from build123d import *

# Parameters (mm, degrees)
ESBO_O4_W                = 84
ESBO_O4_H                = 50
RESSALTO_EXTRUS_O2_DEPTH = 3
CORTE_EXTRUS_O2_REACH    = 50.969
ESBO_O5_W                = 12
ESBO_O5_H                = 3
CORTE_EXTRUS_O4_REACH    = 50.969
ESBO_O6_W                = 3
ESBO_O6_H                = 10
ESBO_O11_W               = 3
ESBO_O11_H               = 10
RESSALTO_EXTRUS_O4_DEPTH = 6


with BuildPart() as part:
    # Esboço4 → Ressalto-extrusão2 (new body)
    with BuildSketch(Plane.XY):
        Rectangle(ESBO_O4_W, ESBO_O4_H)
    extrude(amount=RESSALTO_EXTRUS_O2_DEPTH)

    # Esboço5 → Corte-extrusão2 (cut, up to next)
    with BuildSketch(Plane.XY.offset(3), mode=Mode.PRIVATE) as corte_extrus_o2_sk1:
        with Locations((24, 23.5)):
            Rectangle(ESBO_O5_W, ESBO_O5_H)
    corte_extrus_o2_tool1 = extrude(corte_extrus_o2_sk1.sketch, amount=-CORTE_EXTRUS_O2_REACH, mode=Mode.PRIVATE) & part.part
    # Esboço5 → Corte-extrusão2 (cut, up to next)
    with BuildSketch(Plane.XY.offset(3), mode=Mode.PRIVATE) as corte_extrus_o2_sk2:
        with Locations((-24, 23.5)):
            Rectangle(ESBO_O5_W, ESBO_O5_H)
    corte_extrus_o2_tool2 = extrude(corte_extrus_o2_sk2.sketch, amount=-CORTE_EXTRUS_O2_REACH, mode=Mode.PRIVATE) & part.part
    # Esboço5 → Corte-extrusão2 (cut, up to next)
    with BuildSketch(Plane.XY.offset(3), mode=Mode.PRIVATE) as corte_extrus_o2_sk3:
        with Locations((0, 23.5)):
            Rectangle(ESBO_O5_W, ESBO_O5_H)
    corte_extrus_o2_tool3 = extrude(corte_extrus_o2_sk3.sketch, amount=-CORTE_EXTRUS_O2_REACH, mode=Mode.PRIVATE) & part.part
    # Esboço5 → Corte-extrusão2 (cut, up to next)
    with BuildSketch(Plane.XY.offset(3), mode=Mode.PRIVATE) as corte_extrus_o2_sk4:
        with Locations((0, -23.5)):
            Rectangle(ESBO_O5_W, ESBO_O5_H)
    corte_extrus_o2_tool4 = extrude(corte_extrus_o2_sk4.sketch, amount=-CORTE_EXTRUS_O2_REACH, mode=Mode.PRIVATE) & part.part
    # Esboço5 → Corte-extrusão2 (cut, up to next)
    with BuildSketch(Plane.XY.offset(3), mode=Mode.PRIVATE) as corte_extrus_o2_sk5:
        with Locations((-24, -23.5)):
            Rectangle(ESBO_O5_W, ESBO_O5_H)
    corte_extrus_o2_tool5 = extrude(corte_extrus_o2_sk5.sketch, amount=-CORTE_EXTRUS_O2_REACH, mode=Mode.PRIVATE) & part.part
    # Esboço5 → Corte-extrusão2 (cut, up to next)
    with BuildSketch(Plane.XY.offset(3), mode=Mode.PRIVATE) as corte_extrus_o2_sk6:
        with Locations((24, -23.5)):
            Rectangle(ESBO_O5_W, ESBO_O5_H)
    corte_extrus_o2_tool6 = extrude(corte_extrus_o2_sk6.sketch, amount=-CORTE_EXTRUS_O2_REACH, mode=Mode.PRIVATE) & part.part
    add(corte_extrus_o2_tool1.solids().sort_by_distance((24, 23.5, 3))[0], mode=Mode.SUBTRACT)
    add(corte_extrus_o2_tool2.solids().sort_by_distance((-24, 23.5, 3))[0], mode=Mode.SUBTRACT)
    add(corte_extrus_o2_tool3.solids().sort_by_distance((0, 23.5, 3))[0], mode=Mode.SUBTRACT)
    add(corte_extrus_o2_tool4.solids().sort_by_distance((0, -23.5, 3))[0], mode=Mode.SUBTRACT)
    add(corte_extrus_o2_tool5.solids().sort_by_distance((-24, -23.5, 3))[0], mode=Mode.SUBTRACT)
    add(corte_extrus_o2_tool6.solids().sort_by_distance((24, -23.5, 3))[0], mode=Mode.SUBTRACT)

    # Esboço6 → Corte-extrusão4 (cut, up to next)
    with BuildSketch(Plane.XY, mode=Mode.PRIVATE) as corte_extrus_o4_sk1:
        with Locations((40.5, 10)):
            Rectangle(ESBO_O6_W, ESBO_O6_H)
    corte_extrus_o4_tool1 = extrude(corte_extrus_o4_sk1.sketch, amount=CORTE_EXTRUS_O4_REACH, mode=Mode.PRIVATE) & part.part
    # Esboço6 → Corte-extrusão4 (cut, up to next)
    with BuildSketch(Plane.XY, mode=Mode.PRIVATE) as corte_extrus_o4_sk2:
        with Locations((-40.5, 10)):
            Rectangle(ESBO_O6_W, ESBO_O6_H)
    corte_extrus_o4_tool2 = extrude(corte_extrus_o4_sk2.sketch, amount=CORTE_EXTRUS_O4_REACH, mode=Mode.PRIVATE) & part.part
    # Esboço6 → Corte-extrusão4 (cut, up to next)
    with BuildSketch(Plane.XY, mode=Mode.PRIVATE) as corte_extrus_o4_sk3:
        with Locations((-40.5, -10)):
            Rectangle(ESBO_O6_W, ESBO_O6_H)
    corte_extrus_o4_tool3 = extrude(corte_extrus_o4_sk3.sketch, amount=CORTE_EXTRUS_O4_REACH, mode=Mode.PRIVATE) & part.part
    # Esboço6 → Corte-extrusão4 (cut, up to next)
    with BuildSketch(Plane.XY, mode=Mode.PRIVATE) as corte_extrus_o4_sk4:
        with Locations((40.5, -10)):
            Rectangle(ESBO_O6_W, ESBO_O6_H)
    corte_extrus_o4_tool4 = extrude(corte_extrus_o4_sk4.sketch, amount=CORTE_EXTRUS_O4_REACH, mode=Mode.PRIVATE) & part.part
    add(corte_extrus_o4_tool1.solids().sort_by_distance((40.5, 10, 0))[0], mode=Mode.SUBTRACT)
    add(corte_extrus_o4_tool2.solids().sort_by_distance((-40.5, 10, 0))[0], mode=Mode.SUBTRACT)
    add(corte_extrus_o4_tool3.solids().sort_by_distance((-40.5, -10, 0))[0], mode=Mode.SUBTRACT)
    add(corte_extrus_o4_tool4.solids().sort_by_distance((40.5, -10, 0))[0], mode=Mode.SUBTRACT)

    # Esboço11 → Ressalto-extrusão4 (add)
    with BuildSketch(Plane.ZY.offset(42)):
        with Locations((1.5, 0)):
            Rectangle(ESBO_O11_W, ESBO_O11_H)
        with Locations((1.5, 20)):
            Rectangle(ESBO_O11_W, ESBO_O11_H)
    extrude(amount=RESSALTO_EXTRUS_O4_DEPTH)


solid = part.part
Verification items for the finished model (mm, model axes). A direction names the side the tool comes from. Coordinates: 2 decimals unless noted, no trailing zeros. Loops run counter-clockwise (first coordinate to the right, second up) from the corner with the lowest first, then second, coordinate; pieces in that order, holes last. Notation, with made-up numbers: (73.25, 79) -> (96.25, 79) arc R19 ccw to (96.25, 88) -> close; hole circle Ø6 at (10, 71.5). An arc over 180 degrees is marked (long way). Answer as a JSON object with one key per item and string values. Group by question number.
Item 1: Depth check by flat-ended pin: pin 1 (0.9 mm diameter, centred on y = -9, z = 1, fed in from -X); pin 2 (0.9 mm diameter, centred on x = 3, z = 1.5, fed in from -Y); pin 3 (12 mm diameter, centred on x = 16.5, y = -2, fed in from -Z). Enter the tip coordinate at first touch or a pass-through.
Item 2: Sectioned sample at B-B on x = -1. Record the boundary of the cut face in (y, z), plus the area to 3 significant figures.
Item 3: Scan lines: probe 1 along X at (y, z) = (-7, 1.9); probe 2 along Y at (x, z) = (23, 0.7); probe 3 along X at (y, z) = (-16.5, 0.25). Record each from-to range of solid material in increasing order.
Item 4: Tool access check on faces 4 (the flat face through (-43, 5, 1)), 5 (the flat face through (-18, -24, 2)), 6 (the flat face through (-42, -20, 1)), 7 (the flat face through (-24, 22, 2)). Record the directions out of +Z, -Z, +X, -X, +Y, -Y that give a thin tool (end or side, any length) a straight path to the whole face; none if there is none.
Item 5: Mould release check, pull along Y, two halves, no side actions. Record for faces 1 (the flat face through (24, 22, 2)), 2 (the flat face through (39, 10, 1)), 3 (the flat face through (42, 0, 1)): +Y half, -Y half, draft (parallel to the pull), parting line (faces both ways), or undercut.
Item 6: Sectioned sample at A-A on y = -20. Record the boundary of the cut face in (x, z).
Evaluation:
{
 "1": {"pin 1": "stops at x = -39", "pin 2": "stops at y = -22", "pin 3": "stops at z = 0"},
 "2": {"outline": "(-22, 0) -> (22, 0) -> (22, 3) -> (-22, 3) -> close", "area": "132 mm²"},
 "3": {"probe 1": "x = -39 to 39", "probe 2": "y = -22 to 22", "probe 3": "x = -42 to 42"},
 "4": {"face 4": "+Z, -Z, -X", "face 5": "+Z, -Z, -Y", "face 6": "+Z, -Z, -X, -Y", "face 7": "+Z, -Z, +Y"},
 "5": {"face 1": "+Y half", "face 2": "undercut", "face 3": "draft"},
 "6": {"outline": "(-42, 0) -> (42, 0) -> (42, 3) -> (-42, 3) -> close"}
}
